```python
from build123d import *

# Parameters (mm, degrees)
SKETCH1_W           = 50
SKETCH1_H           = 50
BOSS_EXTRUDE1_DEPTH = 125
SKETCH2_R           = 5
CUT_EXTRUDE1_DEPTH  = 145
SKETCH3_R           = 4
CUT_EXTRUDE2_DEPTH  = 145
CUT_EXTRUDE3_START  = -47
SKETCH4_W           = 44
SKETCH4_H           = 123
SKETCH4_R           = 5
CUT_EXTRUDE3_DEPTH  = 47
SKETCH5_R           = 1
CUT_EXTRUDE4_DEPTH  = 5


with BuildPart() as part:
    # Sketch1 → Boss-Extrude1 (new body)
    with BuildSketch(Plane.XY):
        with Locations((-25, 25)):
            Rectangle(SKETCH1_W, SKETCH1_H)
    extrude(amount=BOSS_EXTRUDE1_DEPTH)

    # Sketch2 → Cut-Extrude1 (cut)
    with BuildSketch(Plane(origin=(0, 50, 0), x_dir=(1, 0, 0), z_dir=(0, 1, 0))):
        with Locations(Location((-25, -17.5, 0), (0, 0, 180))):
            Circle(SKETCH2_R)
        with Locations(Location((-25, -47.5, 0), (0, 0, 180))):
            Circle(SKETCH2_R)
        with Locations(Location((-25, -77.5, 0), (0, 0, 180))):
            Circle(SKETCH2_R)
        with Locations(Location((-25, -107.5, 0), (0, 0, 180))):
            Circle(SKETCH2_R)
    extrude(amount=-CUT_EXTRUDE1_DEPTH, mode=Mode.SUBTRACT)

    # Sketch3 → Cut-Extrude2 (cut)
    with BuildSketch(Plane(origin=(0, 0, 0), x_dir=(-1, 0, 0), z_dir=(0, 0, -1))):
        with Locations((25, 25)):
            Circle(SKETCH3_R)
    extrude(amount=-CUT_EXTRUDE2_DEPTH, mode=Mode.SUBTRACT)

    # Sketch4 → Cut-Extrude3 (cut)
    with BuildSketch(Plane(origin=(0, 0, 0), x_dir=(-1, 0, 0), z_dir=(0, -1, 0)).offset(CUT_EXTRUDE3_START)):
        with Locations((25, -62.5)):
            Rectangle(SKETCH4_W, SKETCH4_H)
        with Locations((25, -47.5)):
            Circle(SKETCH4_R, mode=Mode.SUBTRACT)
        with Locations((25, -107.5)):
            Circle(SKETCH4_R, mode=Mode.SUBTRACT)
        with Locations((25, -77.5)):
            Circle(SKETCH4_R, mode=Mode.SUBTRACT)
        with Locations((25, -17.5)):
            Circle(SKETCH4_R, mode=Mode.SUBTRACT)
    extrude(amount=CUT_EXTRUDE3_DEPTH, mode=Mode.SUBTRACT)

    # Sketch5 → Cut-Extrude4 (cut)
    with BuildSketch(Plane(origin=(0, 0, 0), x_dir=(-1, 0, 0), z_dir=(0, -1, 0))):
        with Locations(Location((48.515610021, -122, 0), (0, 0, 90))):
            Circle(SKETCH5_R)
        with Locations(Location((1.594830842, -122, 0), (0, 0, 90))):
            Circle(SKETCH5_R)
        with Locations(Location((48.515610021, -3, 0), (0, 0, 90))):
            Circle(SKETCH5_R)
        with Locations(Location((1.594830842, -3, 0), (0, 0, 90))):
            Circle(SKETCH5_R)
    extrude(amount=-CUT_EXTRUDE4_DEPTH, mode=Mode.SUBTRACT)


solid = part.part
```
Check sheet for the modelled part. Datum: model origin and axes. Units: mm. A direction names the side the tool comes from. Round coordinates to 2 decimals unless told otherwise and drop trailing zeros. Write each loop counter-clockwise with the first axis right and the second up, starting at its lowest first coordinate (ties: lowest second). Pieces come first, ordered by that corner, then holes. Notation, with made-up numbers: (86.25, 76) -> (111.25, 76) arc R30 cw to (111.25, 111) -> close; hole circle Ø11 at (28.5, 79.25). An arc over 180 degrees is marked (long way). Put each result on its own line as item: value.
(1) Sectioned sample at A-A (x = -25). Count the separate pieces of the cut face and the enclosed holes in it, plus the area to 3 significant figures.
Values found:
separate pieces: 7
enclosed holes: 0
area: 333 mm^2
(2) Mould release check, pull along Y, two halves, no side actions. Record for faces 1 (the face through (-25, 47, 62)), 2 (the face through (-24.479, 28.966, 0.493)), 3 (the face through (-30, 24, 1)): released by +Y, released by -Y, zero draft, split by the parting line, or undercut.
Values found:
face 1: released by -Y
face 2: undercut
face 3: zero draft
(3) Material ranges on line 1 (X direction, y = 1.4, z = 122); line 2 (Z direction, x = -15, y = 14.5); line 3 (Z direction, x = -25, y = 48.5), recorded low to high.
Values found:
line 1: x = -50 to -49.52, -47.52 to -47, -3 to -2.59, -0.59 to 0
line 2: z = 0 to 1, 124 to 125
line 3: z = 0 to 12.5, 22.5 to 42.5, 52.5 to 72.5, 82.5 to 102.5, 112.5 to 125
(4) Go/stop test with flat-tipped pins: pin 1 Ø1.6 at (x, z) = (-48.52, 122) entering from -Y; pin 2 Ø2 at (x, z) = (-6, 29.5) entering from -Y. Record where each tip stops, or that it passes through.
Values found:
pin 1: stops at y = 5
pin 2: stops at y = 47
(5) Sectioned sample at B-B (y = 11). Enter the section's corners in (x, z).
Values found:
outline: (-50, 0) -> (0, 0) -> (0, 125) -> (-50, 125) -> close; hole (-47, 1) -> (-3, 1) -> (-3, 124) -> (-47, 124) -> close
(6) Sectioned sample at D-D (z = 31). Enter the section's corners in (x, y), plus the area to 3 significant figures.
Values found:
outline: (-50, 0) -> (-47, 0) -> (-47, 47) -> (-3, 47) -> (-3, 0) -> (0, 0) -> (0, 50) -> (-50, 50) -> close
area: 432 mm^2
(7) Tool access check on faces 4 (the face through (-25, 50, 62)), 5 (the face through (-47, 24, 63)). Record the directions out of +Z, -Z, +X, -X, +Y, -Y that give a thin tool (end or side, any length) a straight path to the whole face; none if there is none.
Values found:
face 4: +Z, -Z, +X, -X, +Y
face 5: -Y
(8) Sectioned sample at C-C (z = 107.5). Enter the section's corners in (x, y).
Values found:
outline: (-50, 0) -> (-47, 0) -> (-47, 47) -> (-30, 47) -> (-30, 50) -> (-50, 50) -> close; (-20, 47) -> (-3, 47) -> (-3, 0) -> (0, 0) -> (0, 50) -> (-20, 50) -> close
